Autodesk Fusion 360 part; units mm, degrees
sketch "Sketch13" plane through (0, 0, 0) normal (0, 1, 0) x (1, 0, 0)
  line L0 (70, 0) -> (70, 81)
  line L1 (70, 81) -> (15, 81)
  line L2 (15, 81) -> (15, 0)
  line L3 (15, 0) -> (70, 0)
  line L4 (0, 0) -> (121.9113, 0) construction
  dimension "d66" = 55
  dimension "d130" = 81
  dimension "d131" = 15
extrude "Extrude10" add sketch "Sketch13" along normal blind 10
sketch "Sketch14" plane through (0, 10, 0) normal (0, 1, 0) x (-1, 0, 0)
  line L0 (-15, -81) -> (-15, 0)
  line L1 (-70, 0) -> (-70, -81)
  line L2 (-70, -81) -> (-15, -81)
  line L3 (-15, -73.5) -> (-30, -58.5)
  line L4 (-30, -58.5) -> (-30, -22.5)
  line L5 (-30, -22.5) -> (-15, -7.5)
  line L6 (-15, -40.5) -> (-70, -40.5) construction
  line L7 (-42.5, -81) -> (-42.5, 0) construction
  line L8 (-30, -40.5) -> (-87.9308, -40.5) construction
  line L9 (-70, -7.5) -> (-55, -22.5)
  line L10 (-55, -22.5) -> (-55, -58.5)
  line L11 (-55, -58.5) -> (-70, -73.5)
  circle A0 centre (-42.5, -76.5) radius 1.5
  circle A1 centre (-60, -76.5) radius 1.5
  circle A2 centre (-77.5, -76.5) radius 1.5
  circle A3 centre (-25, -76.5) radius 1.5
  circle A4 centre (-7.5, -76.5) radius 1.5
  line L12 (-7.5, -76.5) -> (-77.5, -76.5) construction
  circle A5 centre (-7.5, -4.5) radius 1.5
  circle A6 centre (-25, -4.5) radius 1.5
  circle A7 centre (-42.5, -4.5) radius 1.5
  circle A8 centre (-60, -4.5) radius 1.5
  circle A9 centre (-77.5, -4.5) radius 1.5
  line L13 (-7.5, -4.5) -> (-77.5, -4.5) construction
  line L14 (-15, 0) -> (-70, 0)
  line L15 (-30, -22.5) -> (-15, -22.5)
  line L16 (-55, -22.5) -> (-70, -22.5)
  line L17 (-30, -58.5) -> (-15, -58.5)
  line L18 (-55, -58.5) -> (-70, -58.5)
  line L19 (-70, -58.5) -> (-70, -73.5)
  line L20 (-15, -58.5) -> (-15, -73.5)
  line L21 (-15, -22.5) -> (-15, -7.5)
  line L22 (-70, -22.5) -> (-70, -7.5)
  line L23 (-70, -22.5) -> (-70, -58.5)
  line L24 (-15, -22.5) -> (-15, -58.5)
  dimension "d70" = 15
  dimension "d71" = 15
  dimension "d72" = 15
  dimension "d73" = 7.5
  dimension "d76" = 15
  dimension "d77" = 15
  dimension "d78" = 7.5
  dimension "d79" = 7.5
  dimension "d80" = 15
  dimension "d81" = 15
  dimension "d85" = 17.5
  dimension "d86" = 17.5
  dimension "d87" = 17.5
  dimension "d88" = 17.5
  dimension "d89" = 3
  dimension "d90" = 3
  dimension "d91" = 3
  dimension "d92" = 3
  dimension "d93" = 3
  dimension "d94" = 4.5
  dimension "d95" = 17.5
  dimension "d96" = 17.5
  dimension "d97" = 17.5
  dimension "d98" = 17.5
  dimension "d99" = 3
  dimension "d100" = 3
  dimension "d101" = 3
  dimension "d102" = 3
  dimension "d103" = 3
  dimension "d132" = 7.5
  dimension "d139" = 4.5
  dimension "d140" = 72
  dimension "d141" = 40.5
extrude "Extrude11" cut sketch "Sketch14" against normal blind 10 contours L0 L4 L15 L17 L24 | L0 L5 L15 L21 | L1 L10 L16 L18 L23 | L1 L9 L16 L22
sketch "Sketch16" plane through (0, 10, 0) normal (0, 1, 0) x (-1, 0, 0)
  line L0 (-70, -58.5) -> (-70, -81)
  line L1 (-70, -81) -> (-15, -81)
  line L2 (-15, -81) -> (-15, -58.5)
  line L3 (-30, -58.5) -> (-30, -22.5)
  circle A0 centre (-42.5, -40.5) radius 4
  line L4 (-15, 0) -> (-70, 0)
  line L5 (-70, 0) -> (-70, -7.5)
  line L6 (-55, -22.5) -> (-55, -58.5)
  line L7 (-15, -58.5) -> (-30, -58.5)
  line L8 (-30, -22.5) -> (-15, -7.5)
  line L9 (-15, -7.5) -> (-15, 0)
  line L10 (-70, -7.5) -> (-55, -22.5)
  line L11 (-55, -58.5) -> (-70, -58.5)
  dimension "d83" = 8
extrude "Extrude14" cut sketch "Sketch14" against normal blind 10 contours A6 | A8
sketch "Sketch17" plane through (30, 0, 0) normal (-1, 0, 0) x (0, 0, 1)
  line L0 (-58.5, 0) -> (-22.5, 0)
  line L1 (-22.5, 10) -> (-58.5, 10)
  circle A0 centre (-52.5, 6.35) radius 2
  circle A1 centre (-28.5, 6.35) radius 2
  line L2 (-52.5, 6.35) -> (-28.5, 6.35) construction
  line L3 (-58.5, 10) -> (-58.5, 0)
  line L4 (-22.5, 0) -> (-22.5, 10)
  dimension "d105" = 6.35
  dimension "d106" = 4
  dimension "d107" = 4
  dimension "d108" = 40.5
  dimension "d113" = 24
sketch "Sketch22" plane through (0, 10, 0) normal (0, 1, 0) x (-1, 0, 0)
  circle A0 centre (-60, -4.5) radius 1.5
  circle A1 centre (-25, -4.5) radius 1.5
  line L0 (-70, -58.5) -> (-70, -81)
  line L1 (-70, -81) -> (-15, -81)
  line L2 (-15, -81) -> (-15, -58.5)
  line L3 (-30, -58.5) -> (-30, -22.5)
  spline S0 degree 5 poles (-30, -22.5) (-30.6751, -22.9508) (-31.8982, -23.9212) (-33.3513, -25.5829) (-34.5873, -28.1895) (-35.2819, -31.9804) (-35.49, -36.1444) (-35.514, -40.4999) (-35.4911, -44.8557) (-35.2837, -49.0204) (-34.5894, -52.8118) (-33.353, -55.4184) (-31.8992, -57.0796) (-30.6755, -58.0495) (-30, -58.5) knots 0 0 0 0 0 0 0.1 0.2 0.3 0.4 0.5 0.6 0.7 0.8 0.9 1 1 1 1 1 1
  line L4 (-26.6736, -20.2785) -> (-33.3264, -24.7215)
  line L5 (-33.3277, -56.2805) -> (-26.6723, -60.7195)
  spline S1 degree 5 poles (-55, -22.5) (-54.3243, -22.9503) (-53.092, -23.9257) (-51.6007, -25.6127) (-50.2803, -28.2784) (-49.4997, -32.1312) (-49.3061, -36.2868) (-49.4506, -40.5251) (-49.7869, -44.6606) (-50.3396, -48.5814) (-51.2418, -52.2256) (-52.3883, -54.8952) (-53.5623, -56.7538) (-54.4956, -57.9286) (-55, -58.5) knots 0 0 0 0 0 0 0.1 0.2 0.3 0.4 0.5 0.6 0.7 0.8 0.9 1 1 1 1 1 1
  line L6 (-52.3529, -55.5012) -> (-57.6471, -61.4988)
  line L7 (-58.3285, -20.2817) -> (-51.6715, -24.7183)
  line L8 (-15, 0) -> (-70, 0)
  line L9 (-70, 0) -> (-70, -7.5)
  line L10 (-35.5, -40.5) -> (-49.5, -40.5) construction
  line L11 (-55, -22.5) -> (-55, -58.5)
  line L12 (-15, -58.5) -> (-30, -58.5)
  line L13 (-30, -22.5) -> (-15, -7.5)
  line L14 (-15, -7.5) -> (-15, 0)
  line L15 (-70, -7.5) -> (-55, -22.5)
  line L16 (-55, -58.5) -> (-70, -58.5)
  dimension "d135" = 4
  dimension "d136" = 4
  dimension "d137" = 4
  dimension "d138" = 4
  dimension "d161" = 40.5
  dimension "d162" = 14
  dimension "d163" = 35.5
extrude "Extrude22" add 1 faces at (70, 3.3333, -66) along direction (1, 0, 0) blind 15
extrude "Extrude23" add 1 faces at (15, 3.3333, -73.5) along direction (-1, 0, 0) blind 15
extrude "Extrude24" cut sketch "Sketch14" against normal through all contours A0 | A2 | A4
sketch "Sketch24" plane through (0, 0, 0) normal (0, -1, 0) x (1, 0, 0)
  circle A0 centre (7.5, -76.5) radius 1.5
  circle A1 centre (77.5, -76.5) radius 1.5
  circle A2 centre (42.5, -76.5) radius 1.5
  circle A3 centre (60, -4.5) radius 1.5
  circle A4 centre (25, -4.5) radius 1.5
  line L0 (0, -58.5) -> (0, -81)
  line L1 (0, -81) -> (85, -81)
  line L2 (85, -81) -> (85, -58.5)
  line L3 (70, -7.5) -> (70, 0)
  line L4 (70, 0) -> (15, 0)
  line L5 (15, 0) -> (15, -7.5)
  circle A5 centre (25, -4.5) radius 1.5
  circle A6 centre (60, -4.5) radius 1.5
  circle A7 centre (7.5, -76.5) radius 1.5
  circle A8 centre (42.5, -76.5) radius 1.5
  circle A9 centre (77.5, -76.5) radius 1.5
  circle A10 centre (25, -4.5) radius 3
  circle A11 centre (60, -4.5) radius 3
  circle A12 centre (7.5, -76.5) radius 3
  circle A13 centre (42.5, -76.5) radius 3
  circle A14 centre (77.5, -76.5) radius 3
  line L6 (30, -22.5) -> (30, -58.5)
  line L7 (55, -58.5) -> (55, -22.5)
  line L8 (30, -58.5) -> (0, -58.5)
  line L9 (55, -22.5) -> (70, -7.5)
  line L10 (15, -7.5) -> (30, -22.5)
  line L11 (85, -58.5) -> (55, -58.5)
  dimension "d154" = 6
  dimension "d155" = 6
  dimension "d156" = 6
  dimension "d157" = 6
  dimension "d158" = 6
extrude "Extrude25" cut sketch "Sketch24" against normal blind 3 contours A10 | A11 | A12 | A13 | A14
sketch "Sketch25" plane through (0, 10, 0) normal (0, 1, 0) x (-1, 0, 0)
  circle A0 centre (-7.5, -76.5) radius 1.5
  circle A1 centre (-77.5, -76.5) radius 1.5
  circle A2 centre (-42.5, -76.5) radius 1.5
  circle A3 centre (-25, -4.5) radius 1.5
  circle A4 centre (-60, -4.5) radius 1.5
  line L0 (-30, -22.5) -> (-15, -7.5)
  line L1 (-15, -7.5) -> (-15, 0)
  line L2 (-15, 0) -> (-70, 0)
  line L3 (-70, 0) -> (-70, -7.5)
  line L4 (-70, -7.5) -> (-55, -22.5)
  line L5 (-55, -22.5) -> (-55, -58.5)
  line L6 (-55, -58.5) -> (-85, -58.5)
  line L7 (-85, -58.5) -> (-85, -81)
  line L8 (-85, -81) -> (0, -81)
  line L9 (0, -81) -> (0, -58.5)
  line L10 (0, -58.5) -> (-30, -58.5)
  line L11 (-30, -58.5) -> (-30, -22.5)
  line L12 (-30, -58.5) -> (0, -73.5)
  line L13 (-55, -58.5) -> (-85, -73.5)
  line L14 (0, -73.5) -> (0, -58.5)
  line L15 (-30, -58.5) -> (0, -58.5)
  line L16 (-85, -58.5) -> (-85, -73.5)
  line L17 (-55, -58.5) -> (-85, -58.5)
  dimension "d165" = 7.5
  dimension "d166" = 7.5
extrude "Extrude26" cut sketch "Sketch25" against normal blind 10 contours L9 L10 L12 L14 L15 | L6 L7 L13 L16 L17
fillet "Fillet1" radius 10 4 edges at (30, 5, -58.5) (30, 5, -22.5) (55, 5, -58.5) (55, 5, -22.5)
equation "d105 = ( 12.7 / 2 ) * 1 mm"
equation "d108 = ( 81 / 2 ) * 1 mm"
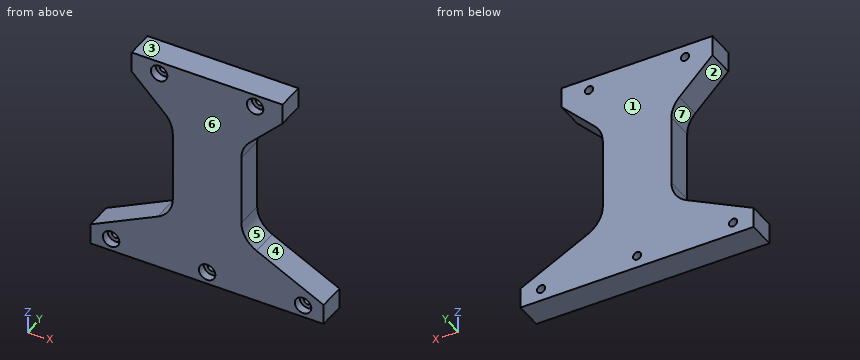
Design review of the part built by this model. Coordinates are the model's own, in mm. Face numbers are marked on the shaded views. A direction names the side the tool comes from. Coordinates: 2 decimals unless noted, no trailing zeros. Loops run counter-clockwise (first coordinate to the right, second up) from the corner with the lowest first, then second, coordinate; pieces in that order, holes last.
Item 1: Wall thickness on L1, parallel to X at y = 5.75, z = -76.5; L2, parallel to Z at x = 25, y = 1.3; L3, parallel to X at y = 1.5, z = -42: over which ranges is each line inside the solid? List them lowest first.
Completed:
L1: x = 0 to 6, 9 to 41, 44 to 76, 79 to 85
L2: z = -81 to -60.98, -17.5 to -7.5, -1.5 to 0
L3: x = 30 to 55
Item 2: Add section A-A (x = 42.5). Write out the cut boundary in (y, z).
Completed:
outline: (0, -81) - (10, -81) - (10, -78) - (3, -78) - (3, -79.5) - (0, -79.5) - close; (0, -73.5) - (3, -73.5) - (3, -75) - (10, -75) - (10, 0) - (0, 0) - close
Item 3: Clearance check with flat-ended pins moving along their axes: pin 1 (5 mm diameter, centred on y = 5.5, z = -37, fed in from +X); pin 2 (1.8 mm diameter, centred on x = 77, z = -75.5, fed in from -Y). State where each tip first meets the part, or that it passes through.
Completed:
pin 1: stops at x = 55
pin 2: stops at y = 3
Item 4: For the marked faces 5, 6 and 7, list the 3-axis set-ups (+Z, -Z, +X, -X, +Y, -Y) from which the entire face can be reached by the end or side of a thin tool; tool diameter is ignored.
Completed:
face 5: +X, +Y, -Y
face 6: +Z, -Z, +X, -X, -Y
face 7: -X, +Y, -Y
Item 5: Add section B-B (z = -4.5). Write out the cut boundary in (x, y).
Completed:
outline: (15, 0) - (22, 0) - (22, 3) - (23.5, 3) - (23.5, 10) - (15, 10) - close; (26.5, 3) - (28, 3) - (28, 0) - (57, 0) - (57, 3) - (58.5, 3) - (58.5, 10) - (26.5, 10) - close; (61.5, 3) - (63, 3) - (63, 0) - (70, 0) - (70, 10) - (61.5, 10) - close
Item 6: Draft analysis for pull direction Z (two halves, no side actions). For the marked faces 1, 2, 3 and 4, state which applies: pulls with the +Z half, pulls with the -Z half, needs draft (parallel to the pull), parting line crosses it, or undercut.
Completed:
face 1: needs draft
face 2: undercut
face 3: pulls with the +Z half
face 4: undercut
Item 7: Add section C-C (y = 2). Write out the cut boundary in (x, z).
Completed:
outline: (0, -81) - (85, -81) - (85, -73.5) - (60.53, -61.26) arc R10 cw to (55, -52.32) - (55, -26.64) arc R10 cw to (57.93, -19.57) - (70, -7.5) - (70, 0) - (15, 0) - (15, -7.5) - (27.07, -19.57) arc R10 cw to (30, -26.64) - (30, -52.32) arc R10 cw to (24.47, -61.26) - (0, -73.5) - close; hole circle Ø6 at (7.5, -76.5); hole circle Ø6 at (25, -4.5); hole circle Ø6 at (42.5, -76.5); hole circle Ø6 at (60, -4.5); hole circle Ø6 at (77.5, -76.5)
Item 8: Add section D-D (x = 77.5). Write out the cut boundary in (y, z).
Completed:
outline: (0, -81) - (10, -81) - (10, -78) - (3, -78) - (3, -79.5) - (0, -79.5) - close; (0, -73.5) - (3, -73.5) - (3, -75) - (10, -75) - (10, -69.75) - (0, -69.75) - close
